Can you work these out from the model? Positions are in its coordinate system, mm. Face numbers are marked on the shaded views. A direction names the side the tool comes from. Coordinates: 2 decimals unless noted, no trailing zeros. Loops run counter-clockwise (first coordinate to the right, second up) from the corner with the lowest first, then second, coordinate; pieces in that order, holes last. Notation, with made-up numbers: M 3.25,13 L 54.25,13 A7 cw 54.25,17 Z; hole C 28,42 d3. An arc over 180 degrees is marked long. Return JSON: item names as keys, results as strings. Group by question number.
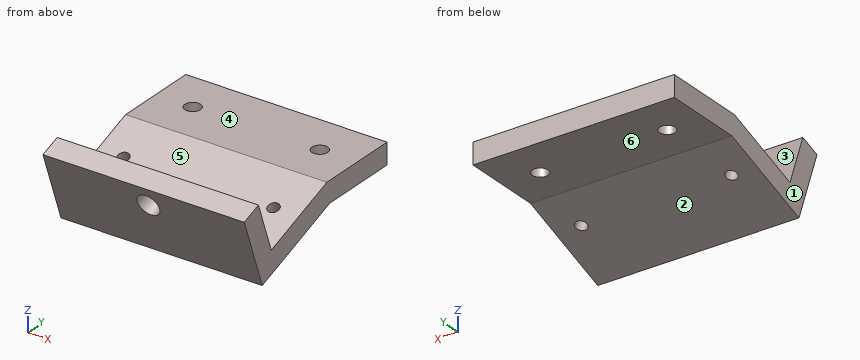
```python
from build123d import *

# Parameters (mm, degrees)
BOSS_EXTRUDE1_DEPTH            = 30.1625
F_1_4_CLEARANCE_HOLE1_D        = 6.7564
M3_CLEARANCE_HOLE1_D           = 3.4
F_3_16_0_1875_DIAMETER_HOLE2_D = 4.7625


with BuildPart() as part:
    # Sketch2 → Boss-Extrude1 (new, symmetric)
    with BuildSketch(Plane(origin=(0, 0, 0), x_dir=(0, 0, -1), z_dir=(1, 0, 0))):
        Polygon((0, 0), (0, 25.4), (6.35, 25.4), (6.35, 1.119676327), (16.689379635, -27.287535752), (-4.195288862, -34.888933437), (-6.367116772, -28.921885295), (8.550503583, -23.49231552), align=None)
    extrude(amount=BOSS_EXTRUDE1_DEPTH, both=True)

    # 1/4 Clearance Hole1 (through all)
    with Locations(Plane(origin=(0, -23.49231552, -8.550503583), x_dir=(1, 0, 0), z_dir=(0, 0.9396926207859081, 0.3420201433256697))):
        with Locations((0, -10)):
            Hole(F_1_4_CLEARANCE_HOLE1_D / 2)

    # M3 Clearance Hole1 (through all)
    with Locations(Plane(origin=(0, 0, 0), x_dir=(1, 0, 0), z_dir=(0, -0.3420201433256693, 0.9396926207859083))):
        with Locations((-22.5, -12.5), (22.5, -12.5)):
            Hole(M3_CLEARANCE_HOLE1_D / 2)

    # 3/16 (0.1875) Diameter Hole2 (through all)
    with Locations(Plane.XY):
        with Locations((-19.05, 12.7), (19.05, 12.7)):
            Hole(F_3_16_0_1875_DIAMETER_HOLE2_D / 2)


solid = part.part
```
1) If I drill on line 1 (Z direction, x = 12, y = 21); line 2 (Z direction, x = 26, y = -15); line 3 (Y direction, x = 4, z = 3.5), over which ranges is the centre line in solid material (lowest first)? Write a range as from..to.
2) For pin 1 (1 mm diameter, centred on x = 13, y = -20.5, fed in from +Z); pin 2 (10 mm diameter, centred on x = 17, y = -0.5, fed in from +Z); pin 3 (8 mm diameter, centred on x = 4, y = 6, fed in from -Z), each with a flat end and sliding along its axis, tell me the tip position at first contact or that it passes through.
3) If we mould it in two halves opening along Y, with no side actions, what happens to the marked faces 1, 2 and 3? For each: +Y half, -Y half, draft (parallel to the pull), parting line (faces both ways), or undercut.
4) Suppose I cut it at D-D, the plane y = -2. List the corners of the cut face in (x, z) for me.
5) Suppose I cut it at A-A, the plane x = 19.05. List the corners of the cut face in (y, z) for me, then the cut area to 3 significant figures.
6) For the marked faces 4, 5 and 6, which set-ups out of +Z, -Z, +X, -X, +Y, -Y let a thin tool reach every point of the face, with its end or its side?
7) Suppose I cut it at B-B, the plane y = 12.7. List the corners of the cut face in (x, z) for me.
8) Suppose I cut it at C-C, the plane x = 0. List the corners of the cut face in (y, z) for me.
Returned:
{
 "1": {"line 1": "z = -6.35..0", "line 2": "z = -12.22..-5.46", "line 3": "y = -34.64..-27.88"},
 "2": {"pin 1": "stops at z = -7.28", "pin 2": "stops at z = 0", "pin 3": "stops at z = -6.35"},
 "3": {"face 1": "draft", "face 2": "+Y half", "face 3": "undercut"},
 "4": {"outline": "M -30.16,-7.49 L 30.16,-7.49 L 30.16,-0.73 L -30.16,-0.73 Z"},
 "5": {"outline": "M -34.89,4.2 L -27.29,-16.69 L 1.12,-6.35 L 10.32,-6.35 L 10.32,0 L 0,0 L -23.49,-8.55 L -28.92,6.37 Z; M 15.08,-6.35 L 25.4,-6.35 L 25.4,0 L 15.08,0 Z", "area": "424 mm²"},
 "6": {"face 4": "+Z, +X, -X, +Y", "face 5": "+Z, +X, -X", "face 6": "-Z, +X, -X, +Y"},
 "7": {"outline": "M -30.16,-6.35 L -21.43,-6.35 L -21.43,0 L -30.16,0 Z; M -16.67,-6.35 L 16.67,-6.35 L 16.67,0 L -16.67,0 Z; M 21.43,-6.35 L 30.16,-6.35 L 30.16,0 L 21.43,0 Z"},
 "8": {"outline": "M -34.89,4.2 L -34.03,1.85 L -28.07,4.02 L -28.92,6.37 Z; M -31.72,-4.5 L -27.29,-16.69 L 1.12,-6.35 L 25.4,-6.35 L 25.4,0 L 0,0 L -23.49,-8.55 L -25.76,-2.33 Z"}
}
